from build123d import *

# Parameters (mm, degrees)
BOSS_EXTRUDE1_DEPTH = 0.9


with BuildPart() as part:
    # Sketch2 → Boss-Extrude1 (new body)
    with BuildSketch(Plane.XY):
        with BuildLine():
            Line((-20.5, -0.4), (-13.5, -0.4))
            ThreePointArc((-13.5, -0.4), (-12.510050506, 0.010050506), (-12.1, 1))
            Line((-12.1, 1), (-12.1, 7))
            ThreePointArc((-12.1, 7), (-11, 8.1), (-9.9, 7))
            Line((-9.9, 7), (-9.9, 0))
            Line((-9.9, 0), (-9.9, -7))
            ThreePointArc((-9.9, -7), (-8, -8.9), (-6.1, -7))
            Line((-6.1, -7), (-6.1, 0))
            Line((-6.1, 0), (-6.1, 7))
            ThreePointArc((-6.1, 7), (-5, 8.1), (-3.9, 7))
            Line((-3.9, 7), (-3.9, 0))
            Line((-3.9, 0), (-3.9, -7))
            ThreePointArc((-3.9, -7), (-2, -8.9), (-0.1, -7))
            Line((-0.1, -7), (-0.1, 0))
            Line((-0.1, 0), (-0.1, 7))
            ThreePointArc((-0.1, 7), (1, 8.1), (2.1, 7))
            Line((2.1, 7), (2.1, 0))
            Line((2.1, 0), (2.1, -7))
            ThreePointArc((2.1, -7), (4, -8.9), (5.9, -7))
            Line((5.9, -7), (5.9, -1))
            ThreePointArc((5.9, -1), (6.075735931, -0.575735931), (6.5, -0.4))
            Line((6.5, -0.4), (13.5, -0.4))
            ThreePointArc((13.5, -0.4), (13.9, 0), (13.5, 0.4))
            Line((13.5, 0.4), (6.5, 0.4))
            ThreePointArc((6.5, 0.4), (5.510050506, -0.010050506), (5.1, -1))
            Line((5.1, -1), (5.1, -7))
            ThreePointArc((5.1, -7), (4, -8.1), (2.9, -7))
            Line((2.9, -7), (2.9, 0))
            Line((2.9, 0), (2.9, 7))
            ThreePointArc((2.9, 7), (1, 8.9), (-0.9, 7))
            Line((-0.9, 7), (-0.9, 0))
            Line((-0.9, 0), (-0.9, -7))
            ThreePointArc((-0.9, -7), (-2, -8.1), (-3.1, -7))
            Line((-3.1, -7), (-3.1, 0))
            Line((-3.1, 0), (-3.1, 7))
            ThreePointArc((-3.1, 7), (-5, 8.9), (-6.9, 7))
            Line((-6.9, 7), (-6.9, 0))
            Line((-6.9, 0), (-6.9, -7))
            ThreePointArc((-6.9, -7), (-8, -8.1), (-9.1, -7))
            Line((-9.1, -7), (-9.1, 0))
            Line((-9.1, 0), (-9.1, 7))
            ThreePointArc((-9.1, 7), (-11, 8.9), (-12.9, 7))
            Line((-12.9, 7), (-12.9, 1))
            ThreePointArc((-12.9, 1), (-13.075735931, 0.575735931), (-13.5, 0.4))
            Line((-13.5, 0.4), (-20.5, 0.4))
            ThreePointArc((-20.5, 0.4), (-20.9, 0), (-20.5, -0.4))
        make_face()
    extrude(amount=BOSS_EXTRUDE1_DEPTH)

    # Sketch3 → Revolve1 (revolve)
    with BuildSketch(Plane(origin=(0, 0, 0), x_dir=(1, 0, 0), z_dir=(0, 1, 0)), mode=Mode.PRIVATE) as revolve1_sk:
        Polygon((-20.5, -0.9), (-25.5, -0.9), (-26.5, 3.1), (-26.5, 29.1), (-20.5, 29.1), align=None)
    revolve(revolve1_sk.sketch.rotate(Axis((-20.5, 0, 0.9), (0, 0, -1)), 175.411434264), axis=Axis((-20.5, 0, 0.9), (0, 0, -1)))

    # Sketch4 → Revolve2 (revolve)
    with BuildSketch(Plane(origin=(0, 0, 0), x_dir=(1, 0, 0), z_dir=(0, 1, 0)), mode=Mode.PRIVATE) as revolve2_sk:
        Polygon((13.5, -0.9), (18.5, -0.9), (19.5, 3.1), (19.5, 29.1), (13.5, 29.1), align=None)
    revolve(revolve2_sk.sketch.rotate(Axis((13.5, 0, 0.9), (0, 0, -1)), 175.609427397), axis=Axis((13.5, 0, 0.9), (0, 0, -1)))


solid = part.part
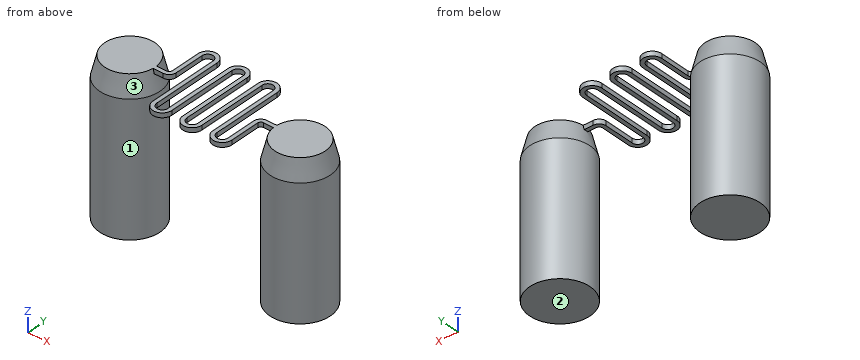
Model file for the job. Use its own axes, mm. Face numbers are marked on the shaded views. Give positions to 0.01 mm unless a question says otherwise; leave off trailing zeros. Order: outer loops, then holes, each group sorted by start corner. A loop starts at its lowest first (then second) coordinate and runs counter-clockwise, first axis right, second up. Notation, with made-up numbers: (74, 34) - (99, 34) arc R34 ccw to (99, 64) - close; hole circle Ø3 at (42.25, -37.75). An arc over 180 degrees is marked (long way). One line per item, written item: value.
Item 1: Slice it at A-A (x = -20.5). List the corners of the cut face in (y, z), then the cut area to 3 significant figures.
Response values:
outline: (-6, -29.1) - (6, -29.1) - (6, -3.1) - (5, 0.9) - (-5, 0.9) - (-6, -3.1) - close
area: 356 mm2
Item 2: Slice it at C-C (z = -13.5). List the corners of the cut face in (x, y).
Response values:
outline: circle Ø12 at (-20.5, 0); circle Ø12 at (13.5, 0)
Item 3: Slice it at B-B (y = 2.5). Give the number of separate pieces and of enclosed holes in the cut face, then the cut area to 3 significant figures.
Response values:
separate pieces: 8
enclosed holes: 0
area: 650 mm2
Item 4: Wall check: line 1 (X direction, y = -0.25, z = -5); line 2 (Y direction, x = -20.5, z = -15.5); line 3 (X direction, y = 3.5, z = -17). Give the ranges that are in metal, low to high.
Response values:
line 1: -26.49 to -14.51, 7.51 to 19.49
line 2: -6 to 6
line 3: -25.37 to -15.63, 8.63 to 18.37
Item 5: Slice it at D-D (x = 1). List the corners of the cut face in (y, z), then the cut area to 3 significant figures.
Response values:
outline: (8.1, 0) - (8.9, 0) - (8.9, 0.9) - (8.1, 0.9) - close
area: 0.720 mm2
Item 6: Pin check, flat tips, straight feed: pin 1 Ø3 at (x, z) = (-14.5, -23.5) entering from -Y; pin 2 Ø0.7 at (y, z) = (1.5, 0.5) entering from -X; pin 3 Ø1 at (y, z) = (3, 0.5) entering from -X. Stop position of each tip, or through.
Response values:
pin 1: y = -3.97
pin 2: x = -25.51
pin 3: x = -24.98
Item 7: Two-plate mould, pull along X, no slides. Class the marked faces 1, 2 and 3: released by +X, released by -X, zero draft, split by the parting line, or undercut.
Response values:
face 1: undercut
face 2: zero draft
face 3: undercut
